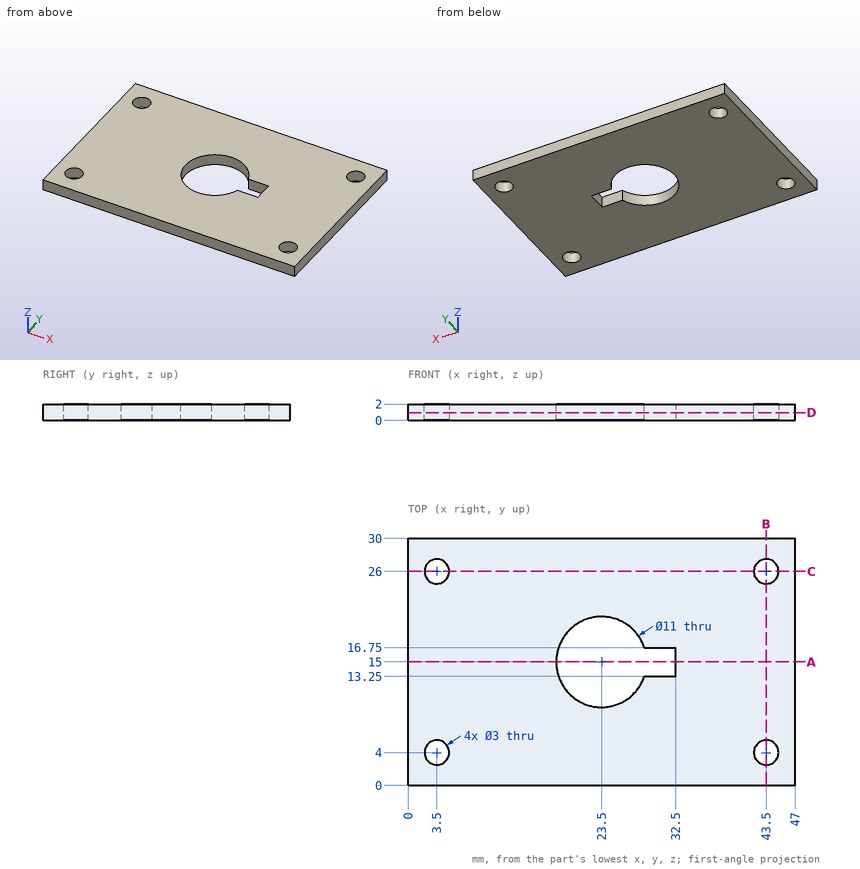
Job drawing, mm, ordinate dimensions from the low corner. One solid piece. Give positions to 0.01 mm unless a question says otherwise; leave off trailing zeros. Loops run counter-clockwise (first coordinate to the right, second up) from the corner with the lowest first, then second, coordinate; pieces in that order, holes last. Notation, with made-up numbers: (81, 74.25) -> (136, 74.25) arc R20 ccw to (136, 79.25) -> close; hole circle Ø11 at (47.5, 18.5). An arc over 180 degrees is marked (long way). Write each question's results on one line, items separated by ' | '. Start each with the question number.
Q1. Band-saw the part on D-D on z = 0.95. List the corners of the cut face in (x, y), plus the area to 3 significant figures.
Q2. Wall check: L1, parallel to Y at x = 43.5, z = 0.9; L2, parallel to Y at x = 23.5, z = 0.55; L3, parallel to X at y = 5, z = 1.65. Give the ranges that are in metal, low to high.
Q3. Pin check, flat tips, straight feed: P1, Ø10, axis at x = 17, y = 18, coming from the -Z side; P2, Ø1.8, axis at x = 3.5, y = 4, coming from the +Z side. Stop position of each tip, or through.
Q4. Band-saw the part on B-B on x = 43.5. List the corners of the cut face in (y, z).
Q5. Band-saw the part on A-A on y = 15. List the corners of the cut face in (x, z).
Q6. Band-saw the part on C-C on y = 26. List the corners of the cut face in (x, z).
Results are:
1) outline: (0, 0) -> (47, 0) -> (47, 30) -> (0, 30) -> close; hole circle Ø3 at (3.5, 4); hole circle Ø3 at (3.5, 26); hole (28.71, 13.25) -> (32.5, 13.25) -> (32.5, 16.75) -> (28.71, 16.75) arc R5.5 ccw (long way) to start; hole circle Ø3 at (43.5, 4); hole circle Ø3 at (43.5, 26) | area: 1,270 mm²
2) L1: y = 0 to 2.5, 5.5 to 24.5, 27.5 to 30 | L2: y = 0 to 9.5, 20.5 to 30 | L3: x = 0 to 2.38, 4.62 to 42.38, 44.62 to 47
3) P1: stops at z = 0 | P2: passes through
4) outline: (0, 0) -> (2.5, 0) -> (2.5, 2) -> (0, 2) -> close; (5.5, 0) -> (24.5, 0) -> (24.5, 2) -> (5.5, 2) -> close; (27.5, 0) -> (30, 0) -> (30, 2) -> (27.5, 2) -> close
5) outline: (0, 0) -> (18, 0) -> (18, 2) -> (0, 2) -> close; (32.5, 0) -> (47, 0) -> (47, 2) -> (32.5, 2) -> close
6) outline: (0, 0) -> (2, 0) -> (2, 2) -> (0, 2) -> close; (5, 0) -> (42, 0) -> (42, 2) -> (5, 2) -> close; (45, 0) -> (47, 0) -> (47, 2) -> (45, 2) -> close
